from build123d import *

# Parameters (mm, degrees)
REVOLVE1_ANGLE           = 180
CUT_EXTRUDE1_DEPTH       = 39.328351126
SHELL1_DEPTH             = 16
SHELL1_2_DEPTH           = 4
EXTRUDE1_REACH           = 40.328
EXTRUDE1_END_RADIUS      = 16
CUT_EXTRUDE2_REACH       = 40.328
EXTRUDE_THIN1_REACH      = 53.192
EXTRUDE_THIN1_END_RADIUS = 15
EXTRUDE_THIN1_START      = -12
SKETCH5_R                = 5.5
SKETCH5_R_2              = 4.5


with BuildPart() as part:
    # Sketch1 → Revolve1 (revolve)
    with BuildSketch(Plane(origin=(0, 0, 0), x_dir=(-1, 0, 0), z_dir=(0, 0, -1))):
        with BuildLine():
            Line((0, 0), (16, 0))
            Line((16, 0), (16, 16))
            ThreePointArc((16, 16), (11.313708499, 27.313708499), (0, 32))
            Line((0, 32), (0, 0))
        make_face()
    revolve(axis=Axis((0, 0, 0), (0, 1, 0)), revolution_arc=REVOLVE1_ANGLE)

    # Sketch2 → Cut-Extrude1 (cut, through all)
    with BuildSketch(Plane.XY.offset(13.75)):
        with BuildLine():
            Line((8.181534086, 5), (8.181534086, 16))
            ThreePointArc((8.181534086, 16), (0, 24.181534086), (-8.181534086, 16))
            Line((-8.181534086, 16), (-8.181534086, 5))
            Line((-8.181534086, 5), (8.181534086, 5))
        make_face()
    extrude(amount=CUT_EXTRUDE1_DEPTH, mode=Mode.SUBTRACT)

    # Shell1: read off the stored shape, not the designer's step
    # Shell1 outline → Shell1 (cut)
    with BuildSketch(Plane(origin=(0, 0, 0), x_dir=(1, 0, 0), z_dir=(0, 1, 0))):
        with BuildLine():
            ThreePointArc((7.901740315, -12.75), (13.105840391, -7.296365372), (15, 0))
            Line((15, 0), (-15, 0))
            ThreePointArc((-15, 0), (-13.105840391, -7.296365372), (-7.901740315, -12.75))
            Line((-7.901740315, -12.75), (7.901740315, -12.75))
        make_face()
    extrude(amount=SHELL1_DEPTH, mode=Mode.SUBTRACT)

    # Shell1 2 outline → Shell1 2 (cut)
    with BuildSketch(Plane(origin=(0, 0, 0), x_dir=(1, 0, 0), z_dir=(0, 1, 0))):
        with BuildLine():
            ThreePointArc((-7.901740315, -12.75), (0, -15), (7.901740315, -12.75))
            Line((7.901740315, -12.75), (-7.901740315, -12.75))
        make_face()
    extrude(amount=SHELL1_2_DEPTH, mode=Mode.SUBTRACT)

    # Shell1 3 outline → Shell1 3 (revolve, cut)
    with BuildSketch(Plane.XZ.offset(-16)):
        with BuildLine():
            ThreePointArc((15, 0), (13.105840391, 7.296365372), (7.901740315, 12.75))
            Line((7.901740315, 12.75), (0, 12.75))
            Line((0, 12.75), (0, 0))
            Line((0, 0), (15, 0))
        make_face()
    revolve(axis=Axis((0, 16, 0), (0, 0, 1)), mode=Mode.SUBTRACT)

    # Extrude1: up to this cylinder (the profile starts inside it)
    extrude1_end = Plane(origin=(0, 6.31611, 0), z_dir=(0, -1, 0)) * Cylinder(EXTRUDE1_END_RADIUS, 113.656, mode=Mode.PRIVATE)
    # Sketch3 → Extrude1 (add, up to the surface)
    with BuildSketch(Plane.XY.offset(13.75), mode=Mode.PRIVATE) as extrude1_sk1:
        with BuildLine():
            Line((6.076328446, 7.830430308), (8.181534086, 5))
            Line((8.181534086, 5), (-8.181534086, 5))
            Line((-8.181534086, 5), (-6.076328446, 7.830430308))
            ThreePointArc((-6.076328446, 7.830430308), (0, 5.818465914), (6.076328446, 7.830430308))
        make_face()
    extrude1_tool1 = extrude(extrude1_sk1.sketch, amount=EXTRUDE1_REACH, mode=Mode.PRIVATE) & extrude1_end
    add(extrude1_tool1.solids().sort_by_distance((6.995686, 6.31611, 13.75))[0])

    # Sketch4 → Cut-Extrude2 (cut, up to next)
    with BuildSketch(Plane.XY.offset(13.75), mode=Mode.PRIVATE) as cut_extrude2_sk1:
        Polygon((-3.535533906, 16), (0, 12.464466094), (3.535533906, 16), (0, 19.535533906), align=None)
    cut_extrude2_tool1 = extrude(cut_extrude2_sk1.sketch, amount=-CUT_EXTRUDE2_REACH, mode=Mode.PRIVATE) & part.part
    add(cut_extrude2_tool1.solids().sort_by_distance((0, 16, 13.75))[0], mode=Mode.SUBTRACT)

    # Mirror1: part across face


with BuildPart() as part_1:
    add(part.part)
    add(part.part.mirror(Plane(origin=(0, 18.784156894, 0), x_dir=(1, 0, 0), z_dir=(0, 0, -1))))

    # Extrude-Thin1: up to this sphere (the profile starts inside it)
    extrude_thin1_end = Location((0, 16, 0)) * Sphere(EXTRUDE_THIN1_END_RADIUS, mode=Mode.PRIVATE)
    # Sketch5 → Extrude-Thin1 (add, up to the surface)
    with BuildSketch(Plane.XZ.offset(EXTRUDE_THIN1_START), mode=Mode.PRIVATE) as extrude_thin1_sk1:
        Circle(SKETCH5_R)
        Circle(SKETCH5_R_2, mode=Mode.SUBTRACT)
    extrude_thin1_tool1 = extrude(extrude_thin1_sk1.sketch, amount=-EXTRUDE_THIN1_REACH, mode=Mode.PRIVATE) & extrude_thin1_end
    add(extrude_thin1_tool1.solids().sort_by_distance((-5.344437, 12, 0))[0])


solid = part_1.part
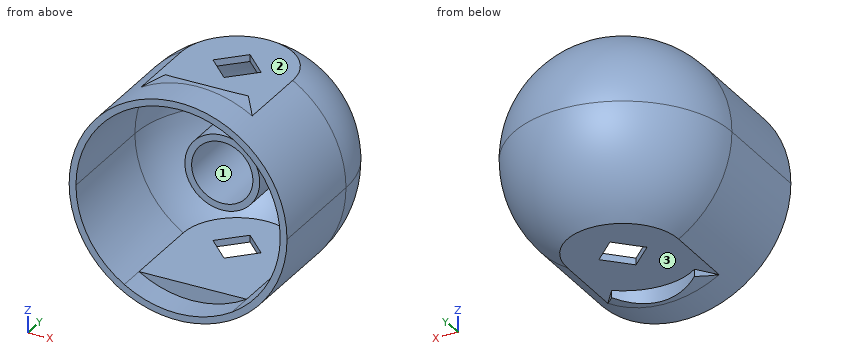
Input: part model. Units: mm. Frame: model coordinates. Face numbers are marked on the shaded views. Give positions to 0.01 mm unless a question says otherwise; leave off trailing zeros. Order: outer loops, then holes, each group sorted by start corner. A loop starts at its lowest first (then second) coordinate and runs counter-clockwise, first axis right, second up.
Q1. Section B-B on x = 2.5. State how many separate pieces and enclosed holes the cut face has, and give its area (3 significant figures).
Checked values:
separate pieces: 3
enclosed holes: 0
area: 126 mm2
Q2. Section A-A on y = 9. Output: boundary loops of the cut face in (x, z), and give its area (3 significant figures).
Checked values:
outline: (-8.18, -13.75) - (8.18, -13.75) arc R16 ccw to (8.18, 13.75) - (-8.18, 13.75) arc R16 ccw to start; hole (-7.9, -12.75) - (7.9, -12.75) arc R15 ccw to (7.9, 12.75) - (-7.9, 12.75) arc R15 ccw to start
area: 95.7 mm2
Q3. Ray query, probe 1 along X at (y, z) = (15.75, 0); probe 2 along Z at (x, y) = (0, 21); probe 3 along Z at (x, y) = (6, 16). Return the intervals inside material, ascending.
Checked values:
probe 1: x = -16 to -15, -5.5 to -4.5, 4.5 to 5.5, 15 to 16
probe 2: z = -13.75 to -12.75, -5.5 to -4.5, 4.5 to 5.5, 12.75 to 13.75
probe 3: z = -13.75 to -12.75, 12.75 to 13.75
Q4. Draft query along Z for the marked faces 1, 2 and 3. Return one class per face: +Z half, -Z half, draft (parallel to the pull), parting line (faces both ways), or undercut.
Checked values:
face 1: undercut
face 2: +Z half
face 3: -Z half
Q5. Section D-D on y = 25. Output: boundary loops of the cut face in (x, z).
Checked values:
outline: circle Ø26.46 at (0, 0); circle Ø11 at (0, 0); hole circle Ø24 at (0, 0); hole circle Ø9 at (0, 0)
Q6. Contact query for flat-ended pins moving along their axis: pin 1 Ø13 at (x, y) = (-4, 18) entering from -Z; pin 2 Ø1.5 at (x, y) = (-7.5, 21) entering from -Z; pin 3 Ø0.7 at (x, z) = (-1.5, -13.5) entering from -Y; pin 4 Ø8 at (y, z) = (7.5, 4) entering from +X. Output: stop coordinate, or through.
Checked values:
pin 1: stops at z = -13.75
pin 2: stops at z = -13.7
pin 3: stops at y = 4
pin 4: stops at x = 16
Q7. Section C-C on y = 13. Output: boundary loops of the cut face in (x, z), and give its area (3 significant figures).
Checked values:
outline: (-8.18, -13.75) - (-0.54, -13.75) - (-0.54, -12.75) - (-7.9, -12.75) arc R15 cw to (-7.9, 12.75) - (-0.54, 12.75) - (-0.54, 13.75) - (-8.18, 13.75) arc R16 ccw to start; circle Ø11 at (0, 0); (0.54, -13.75) - (8.18, -13.75) arc R16 ccw to (8.18, 13.75) - (0.54, 13.75) - (0.54, 12.75) - (7.9, 12.75) arc R15 cw to (7.9, -12.75) - (0.54, -12.75) - close; hole circle Ø9 at (0, 0)
area: 125 mm2
